Could you check a few things on this drawing? It's one solid part, dimensions in mm from its lowest x, y, z. Give positions to 0.01 mm unless a question says otherwise; leave off trailing zeros. Order: outer loops, then holes, each group sorted by start corner. A loop starts at its lowest first (then second) coordinate and runs counter-clockwise, first axis right, second up. Notation, with made-up numbers: (28, 76.25) - (64, 76.25) arc R14 cw to (64, 80.25) - close; hole circle Ø11 at (69, -36.75). An arc over 180 degrees is marked (long way). Put each result on its own line as item: value.
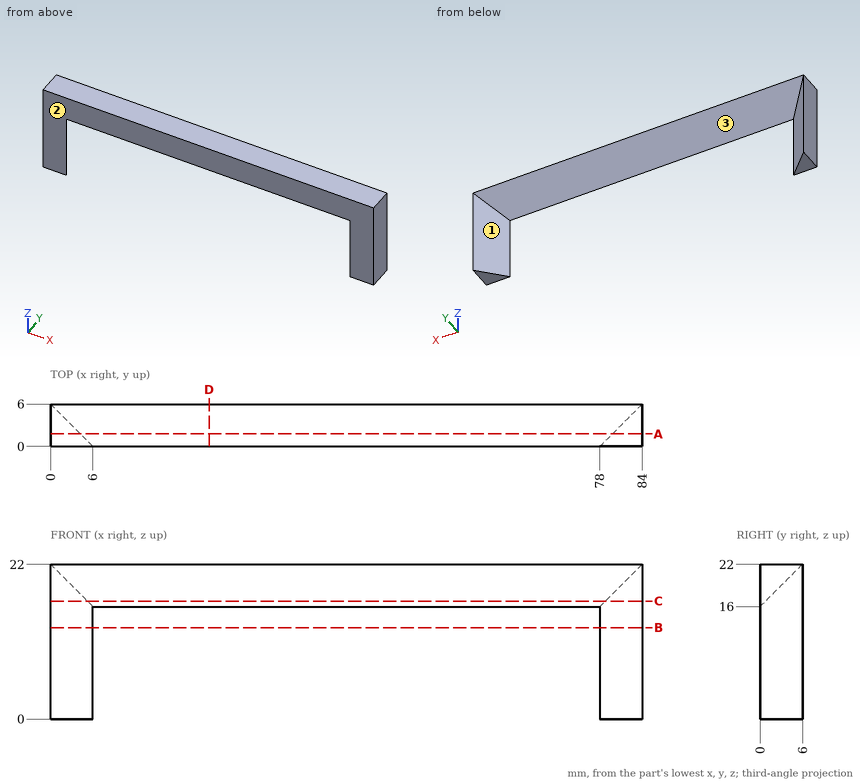
1) Suppose I cut it at B-B, the plane z = 13. List the corners of the cut face in (x, y) for me.
Filled in:
outline: (0, 0) - (6, 0) - (0, 6) - close; (78, 0) - (84, 0) - (84, 6) - close
2) Suppose I cut it at C-C, the plane z = 16.75. List the corners of the cut face in (x, y) for me, and give its area (3 significant figures).
Filled in:
outline: (0, 0) - (84, 0) - (84, 6) - (78.75, 0.75) - (5.25, 0.75) - (0, 6) - close
area: 90.6 mm^2
3) I'm going to push flat-ended pins straight in: pin 1 (1.5 mm diameter, centred on x = 12.5, z = 13.5, fed in from -Y); pin 2 (1.5 mm diameter, centred on x = 61.5, y = 0.5, fed in from -Z); pin 3 (6 mm diameter, centred on x = 21.5, z = 16, fed in from +Y). Where does each tip first touch, or does it pass through?
Filled in:
pin 1: passes through
pin 2: stops at z = 16
pin 3: stops at y = 3
4) Suppose I cut it at A-A, the plane y = 1.75. List the corners of the cut face in (x, z) for me, and give its area (3 significant figures).
Filled in:
outline: (0, 0) - (4.25, 0) - (4.25, 17.75) - (79.75, 17.75) - (79.75, 0) - (84, 0) - (84, 22) - (0, 22) - close
area: 508 mm^2
5) Suppose I cut it at D-D, the plane x = 22.5. List the corners of the cut face in (y, z) for me, and give its area (3 significant figures).
Filled in:
outline: (0, 16) - (6, 22) - (0, 22) - close
area: 18.0 mm^2
6) We'd pull the mould along X, two halves only. Please class the marked faces 1, 2 and 3: pulls with the +X half, pulls with the -X half, needs draft (parallel to the pull), parting line crosses it, or undercut.
Filled in:
face 1: undercut
face 2: needs draft
face 3: undercut
7) If I drill on line 1 (X direction, y = 0.5, z = 5); line 2 (X direction, y = 4, z = 16.75); line 3 (Z direction, x = 38, y = 1.5), over which ranges is the centre line in solid material (lowest first)? Write a range as [from, to].
Filled in:
line 1: x = [0, 5.5], [78.5, 84]
line 2: x = [0, 2], [82, 84]
line 3: z = [17.5, 22]
